from build123d import *

# Parameters (mm, degrees)
SKETCH1_W                   = 5.334
SKETCH1_H                   = 19.05
M3_5_CLEARANCE_HOLE1_REACH  = 21.654
M3_5_CLEARANCE_HOLE1_BORE_R = 2.0193
M3_5_CLEARANCE_HOLE2_REACH  = 21.654
M3_5_CLEARANCE_HOLE2_BORE_R = 2.0193


with BuildPart() as part:
    # Sketch1 → Revolve1 (revolve)
    with BuildSketch(Plane.XY, mode=Mode.PRIVATE) as revolve1_sk:
        with Locations((2.667, 9.525)):
            Rectangle(SKETCH1_W, SKETCH1_H)
    revolve(revolve1_sk.sketch.rotate(Axis((0, 19.05, 0), (0, -1, 0)), 270), axis=Axis((0, 19.05, 0), (0, -1, 0)))

    # Sketch2 → Hole1 (revolve, cut)
    with BuildSketch(Plane(origin=(0, 0, 0), x_dir=(0, 0, -1), z_dir=(1, 0, 0))):
        Polygon((0, 0), (0, 19.05), (2.5, 19.05), (2.5, 9.930580918), (3.175, 9.525), (3.175, 0), align=None)
    revolve(axis=Axis((0, -6.130023899, 0), (0, 1, 0)), mode=Mode.SUBTRACT)

    # M3.5 Clearance Hole1 bore (on position points) → M3.5 Clearance Hole1 (cut, up to next)
    with BuildSketch(Plane(origin=(0, 15.621, 5.334), x_dir=(1, 0, 0), z_dir=(0, 0, 1)), mode=Mode.PRIVATE) as m3_5_clearance_hole1_sk1:
        Circle(M3_5_CLEARANCE_HOLE1_BORE_R)
    m3_5_clearance_hole1_tool1 = extrude(m3_5_clearance_hole1_sk1.sketch, amount=-M3_5_CLEARANCE_HOLE1_REACH, mode=Mode.PRIVATE) & part.part
    add(m3_5_clearance_hole1_tool1.solids().sort_by_distance((0, 15.621, 5.334))[0], mode=Mode.SUBTRACT)

    # M3.5 Clearance Hole2 bore (on position points) → M3.5 Clearance Hole2 (cut, up to next)
    with BuildSketch(Plane(origin=(0, 3.429, 5.334), x_dir=(1, 0, 0), z_dir=(0, 0, 1)), mode=Mode.PRIVATE) as m3_5_clearance_hole2_sk1:
        Circle(M3_5_CLEARANCE_HOLE2_BORE_R)
    m3_5_clearance_hole2_tool1 = extrude(m3_5_clearance_hole2_sk1.sketch, amount=-M3_5_CLEARANCE_HOLE2_REACH, mode=Mode.PRIVATE) & part.part
    add(m3_5_clearance_hole2_tool1.solids().sort_by_distance((0, 3.429, 5.334))[0], mode=Mode.SUBTRACT)


solid = part.part
Geometry check sheet. Reference: the model listing, model coordinates, mm. A direction names the side the tool comes from. Round coordinates to 2 decimals unless told otherwise and drop trailing zeros. Write each loop counter-clockwise with the first axis right and the second up, starting at its lowest first coordinate (ties: lowest second). Pieces come first, ordered by that corner, then holes. Notation, with made-up numbers: (-20, -15) -> (-1, -15) arc R24 cw to (-1, 5) -> close; hole circle Ø9 at (60, 28). An arc over 180 degrees is marked (long way). One line per item, written item: value. Start each with the question number.
(1) Cross-section at C-C, the plane y = 8.25. Record the cut outline in (x, z) (3 decimals), and give its area (3 significant figures).
(2) Access from +Z, -Z, +X, -X, +Y, -Y to the whole of each face (thin tool, end or side, straight path). Record for faces 1 (the cylindrical face through (-0.95, 4.7, -3.03)), 2 (the cylindrical face through (1.926, 4.036, 3.912)), 3 (the cylindrical face through (-0.751, 14.426, -2.385)).
(3) Scan lines: line 1 (Y direction, x = 0, z = 3.4); line 2 (X direction, y = 4.5, z = 0) (3 decimals); line 3 (X direction, y = 17, z = 0). Record each from-to range of solid material in increasing order. Write a range as [from, to].
(4) Cross-section at B-B, the plane z = 0. Record the cut outline in (x, y) (3 decimals).
(5) Cross-section at A-A, the plane x = 0. Record the cut outline in (y, z) (3 decimals), and give its area (3 significant figures).
(6) Cross-section at D-D, the plane y = 14.25. Record the cut outline in (x, z).
(7) Go/stop test with flat-tipped pins: pin 1 Ø3 at (x, z) = (0, 0) entering from -Y; pin 2 Ø3 at (x, y) = (0, 15.621) entering from +Z; pin 3 Ø3 at (x, y) = (0.5, 15.5) entering from -Z; pin 4 Ø1.5 at (y, z) = (11.5, 2.5) entering from +X. Record where each tip stops, or that it passes through.
(8) Draft check along Y on faces 4 (the flat face through (2.45, 19.05, 1.11)), 5 (the cylindrical face through (1.926, 16.228, 3.431)), 6 (the flat face through (-3.5, 0, -0.1)). Enter one of: +Y half, -Y half, draft (parallel to the pull), parting line (faces both ways), or undercut.
Answer:
1. outline: circle Ø10.668 at (0, 0); hole circle Ø6.35 at (0, 0)
1. area: 57.7 mm²
2. face 1: -Y
2. face 2: +Z
2. face 3: +Y, -Y
3. line 1: [0, 1.41], [5.45, 13.6], [17.64, 19.05]
3. line 2: [-5.334, -3.175], [3.175, 5.334]
3. line 3: [-5.33, -2.5], [2.5, 5.33]
4. outline: (-5.334, 0) -> (-3.175, 0) -> (-3.175, 9.525) -> (-2.5, 9.931) -> (-2.5, 19.05) -> (-5.334, 19.05) -> close; (2.5, 9.931) -> (3.175, 9.525) -> (3.175, 0) -> (5.334, 0) -> (5.334, 19.05) -> (2.5, 19.05) -> close
5. outline: (0, -5.334) -> (19.05, -5.334) -> (19.05, -2.5) -> (9.931, -2.5) -> (9.525, -3.175) -> (0, -3.175) -> close; (0, 3.175) -> (1.41, 3.175) -> (1.41, 5.334) -> (0, 5.334) -> close; (5.448, 3.175) -> (9.525, 3.175) -> (9.931, 2.5) -> (13.602, 2.5) -> (13.602, 5.334) -> (5.448, 5.334) -> close; (17.64, 2.5) -> (19.05, 2.5) -> (19.05, 5.334) -> (17.64, 5.334) -> close
5. area: 74.7 mm²
6. outline: (-1.48, 2.01) -> (-1.48, 5.12) arc R5.33 ccw (long way) to (1.48, 5.12) -> (1.48, 2.01) arc R2.5 cw (long way) to start
7. pin 1: through
7. pin 2: z = -2
7. pin 3: z = -5.33
7. pin 4: x = 5.04
8. face 4: +Y half
8. face 5: undercut
8. face 6: -Y half
